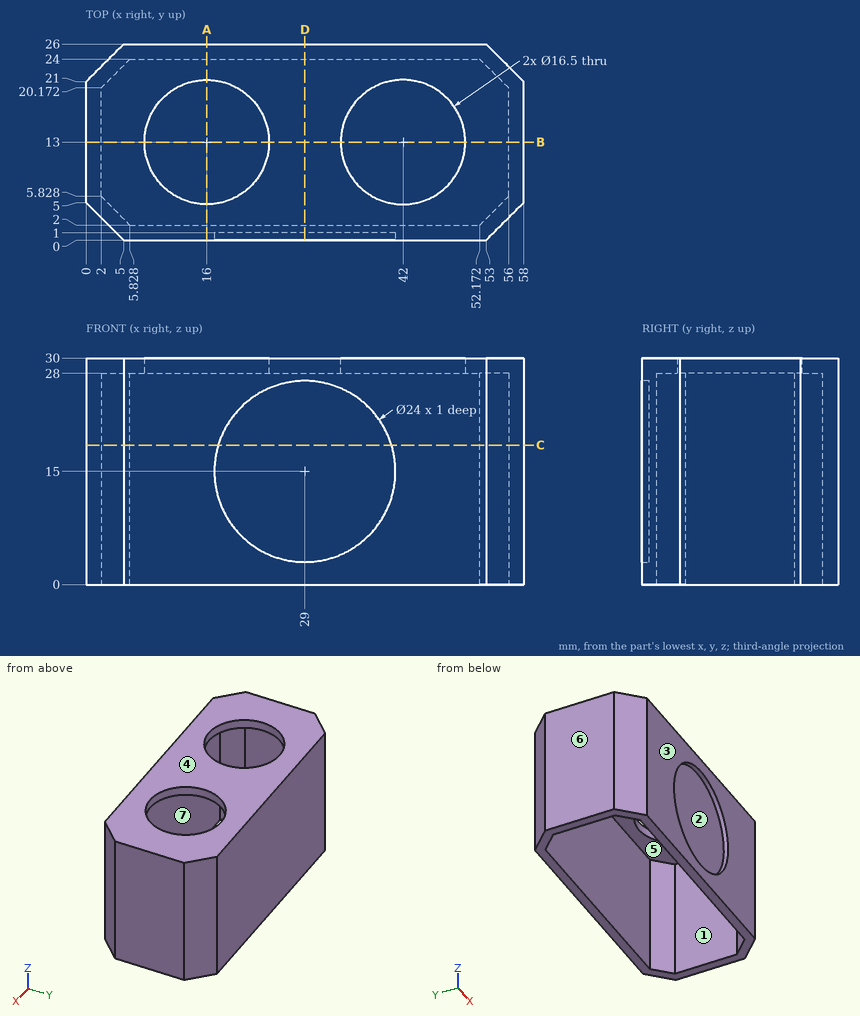
Source: three-view drawing plus pictorial views. Frame: mm from the lowest corner of the part. A direction names the side the tool comes from. Round coordinates to 2 decimals unless told otherwise and drop trailing zeros. Order: outer loops, then holes, each group sorted by start corner. A loop starts at its lowest first (then second) coordinate and runs counter-clockwise, first axis right, second up. Notation, with made-up numbers: (4, 10) - (47, 10) arc R24 ccw to (47, 32) - close; hole circle Ø3 at (49.5, 30). An arc over 180 degrees is marked (long way). Write each question's results on one line, items separated by ' | '.
Item 1: Reachability of the marked faces 1, 2 and 3 from +Z, -Z, +X, -X, +Y, -Y: full face, straight path, thin tool, end or side. Return the list, or none.
Completed:
face 1: -Z | face 2: -Y | face 3: +Z, -Z, +X, -X, -Y
Item 2: Mould query, pull axis X, two halves, no side actions, for the marked faces 4, 5, 6 and 7. Classes: pulls with the +X half, pulls with the -X half, needs draft (parallel to the pull), parting line crosses it, or undercut.
Completed:
face 4: needs draft | face 5: undercut | face 6: pulls with the -X half | face 7: undercut
Item 3: Section D-D, the plane x = 29. Return the cut outline in (y, z), and give its area (3 significant figures).
Completed:
outline: (0, 0) - (2, 0) - (2, 28) - (24, 28) - (24, 0) - (26, 0) - (26, 30) - (0, 30) - (0, 27) - (1, 27) - (1, 3) - (0, 3) - close | area: 140 mm^2
Item 4: Section C-C, the plane z = 18.5. Return the cut outline in (x, y).
Completed:
outline: (0, 5) - (5, 0) - (17.52, 0) - (17.52, 1) - (40.48, 1) - (40.48, 0) - (53, 0) - (58, 5) - (58, 21) - (53, 26) - (5, 26) - (0, 21) - close; hole (2, 5.83) - (5.83, 2) - (52.17, 2) - (56, 5.83) - (56, 20.17) - (52.17, 24) - (5.83, 24) - (2, 20.17) - close
Item 5: Section A-A, the plane x = 16. Return the cut outline in (y, z), and give its area (3 significant figures).
Completed:
outline: (0, 0) - (2, 0) - (2, 28) - (4.75, 28) - (4.75, 30) - (0, 30) - close; (21.25, 28) - (24, 28) - (24, 0) - (26, 0) - (26, 30) - (21.25, 30) - close | area: 131 mm^2
Item 6: Material intervals for line 1 along X through (y, z) = (7.5, 9.75); line 2 along Y through (x, z) = (8.5, 2); line 3 along Y through (x, z) = (42, 29.3), sorted ascending. Write a range as [from, to].
Completed:
line 1: [0, 2], [56, 58] | line 2: [0, 2], [24, 26] | line 3: [0, 4.75], [21.25, 26]
Item 7: Section B-B, the plane y = 13. Return the cut outline in (x, z), and give its area (3 significant figures).
Completed:
outline: (0, 0) - (2, 0) - (2, 28) - (7.75, 28) - (7.75, 30) - (0, 30) - close; (24.25, 28) - (33.75, 28) - (33.75, 30) - (24.25, 30) - close; (50.25, 28) - (56, 28) - (56, 0) - (58, 0) - (58, 30) - (50.25, 30) - close | area: 162 mm^2
